The model under review builds one solid part; all positions refer to its coordinate system, in mm. A direction names the side the tool comes from. Round coordinates to 2 decimals unless told otherwise and drop trailing zeros. Write each loop counter-clockwise with the first axis right and the second up, starting at its lowest first coordinate (ties: lowest second). Pieces come first, ordered by that corner, then holes.
Item 1: To check wall thickness, follow L1, parallel to X at y = -71, z = 66; L2, parallel to Y at x = 66.5, z = 15; L3, parallel to Z at x = -13, y = 63.5. State the ranges of each line that lie inside material, in increasing order.
Item 2: Add section B-B (x = 88). Give the boundary of the cut face in (y, z), plus the area to 3 significant figures.
Item 3: Clearance check with flat-ended pins moving along their axes: pin 1 Ø3 at (x, z) = (101.5, 70.5) entering from +Y; pin 2 Ø3 at (x, y) = (101.5, -36.5) entering from +Z; pin 3 Ø4 at (x, z) = (-59.5, 59.5) entering from +Y. State where each tip first meets the part, or that it passes through.
Item 4: Add section C-C (z = 49). Give the boundary of the cut face in (x, y), plus the area to 3 significant figures.
Item 5: Machinability: for faces 1 (the face through (59.73, -48.19, 1.27)), 2 (the face through (101.871, -55.646, 56.504)), 3 (the face through (98.35, -95.36, 42.96)), which of the approach directions +Z, -Z, +X, -X, +Y, -Y give a long, thin tool a straight path to every point of the face, cutting with its end or side? Answer none if there is none.
Item 6: Add section D-D (y = -19). Give the boundary of the cut face in (x, z), plus the area to 3 significant figures.
Item 7: Draft analysis for pull direction X (two halves, no side actions). For faces 4 (the face through (100.603, -1, 42)), 5 (the face through (-93.89, -19.02, 2.85)), 6 (the face through (100.096, -1.26, 2.852)), state which applies: +X half, -X half, draft (parallel to the pull), parting line (faces both ways), or undercut.
Item 8: Add section A-A (z = 15). Give the boundary of the cut face in (x, y), plus the area to 3 significant figures.
```python
from build123d import *

# Parameters (mm, degrees)
F0_W      = 200
F0_H      = 200
F1_DEPTH  = 75
F2_R      = 10
F3_R      = 50
F4_R      = 10
F5_T      = -2.5
F6_R      = 20.601636
F7_DEPTH  = 200.001
F9_DEPTH  = 2.5
F11_DEPTH = 2.5


with BuildPart() as f1:
    # F0 (on Top) → F1 (new body)
    with BuildSketch(Plane.XY):
        with Locations((3.103165, 0)):
            Rectangle(F0_W, F0_H)
    extrude(amount=F1_DEPTH)

    # F2
    f2_edges = [f1.edges().sort_by_distance(p)[0] for p in [
        (-96.896835, -100, 37.5),
        (103.103165, -100, 37.5),
        (103.103165, 100, 37.5),
    ]]
    fillet(f2_edges, radius=F2_R)

    # F3
    f3_edges = [f1.edges().sort_by_distance(p)[0] for p in [
        (-96.896835, 100, 37.5),
    ]]
    fillet(f3_edges, radius=F3_R)

    # F4
    f4_edges = [f1.edges().sort_by_distance(p)[0] for p in [
        (23.103165, 100, 0),
    ]]
    fillet(f4_edges, radius=F4_R)

    # F5
    f5_openings = [f1.faces().sort_by_distance(p)[0] for p in [
        (4.259549, -1.156383, 75),
    ]]
    offset(amount=F5_T, openings=f5_openings)

    # F6 (on face) → F7 (cut, through all)
    with BuildSketch(Plane.XZ.offset(100)):
        with Locations((0, 44.865675)):
            Circle(F6_R)
    extrude(amount=-F7_DEPTH, mode=Mode.SUBTRACT)

    # F8 (on face) → F9 (cut, through all)
    with BuildSketch(Plane.XY.offset(2.5)):
        with BuildLine():
            ThreePointArc((54.924048, -7.537108), (51.811896, -2.99646), (50.547384, 2.361149))
            ThreePointArc((50.547384, 2.361149), (-39.923575, 29.284524), (14.04054, -48.160533))
            ThreePointArc((14.04054, -48.160533), (21.879419, -48.100018), (28.678354, -52.002092))
            Line((28.678354, -52.002092), (42.298151, -65.621889))
            Line((42.298151, -65.621889), (77.65349, -30.26655))
            Line((77.65349, -30.26655), (54.924048, -7.537108))
        make_face()
    extrude(amount=-F9_DEPTH, mode=Mode.SUBTRACT)

    # F10 (on face) → F11 (cut, through all)
    with BuildSketch(Plane.YZ.offset(103.103165)):
        with BuildLine():
            ThreePointArc((-57.071527, 60), (-55.607061, 56.464466), (-52.071527, 55))
            Line((-52.071527, 55), (-5, 55))
            ThreePointArc((-5, 55), (-1.464466, 56.464466), (0, 60))
            Line((0, 60), (0, 75))
            Line((0, 75), (-57.071527, 75))
            Line((-57.071527, 75), (-57.071527, 60))
        make_face()
    extrude(amount=-F11_DEPTH, mode=Mode.SUBTRACT)


solid = f1.part
```
Numbers:
1. L1: x = -96.9 to -94.4, 100.6 to 103.1
1. L2: y = -100 to -97.5, 97.5 to 100
1. L3: z = 0 to 2.5
2. outline: (-100, 10) arc R10 ccw to (-90, 0) - (90, 0) arc R10 ccw to (100, 10) - (100, 75) - (97.5, 75) - (97.5, 10) arc R7.5 cw to (90, 2.5) - (-90, 2.5) arc R7.5 cw to (-97.5, 10) - (-97.5, 75) - (-100, 75) - close
2. area: 844 mm2
3. pin 1: stops at y = 97.24
3. pin 2: stops at z = 55
3. pin 3: stops at y = 98.86
4. outline: (-96.9, -90) arc R10 ccw to (-86.9, -100) - (-20.18, -100) - (-20.18, -97.5) - (-86.9, -97.5) arc R7.5 cw to (-94.4, -90) - (-94.4, 50) arc R47.5 cw to (-46.9, 97.5) - (-20.18, 97.5) - (-20.18, 100) - (-46.9, 100) arc R50 ccw to (-96.9, 50) - close; (20.18, -100) - (93.1, -100) arc R10 ccw to (103.1, -90) - (103.1, 90) arc R10 ccw to (93.1, 100) - (20.18, 100) - (20.18, 97.5) - (93.1, 97.5) arc R7.5 cw to (100.6, 90) - (100.6, -90) arc R7.5 cw to (93.1, -97.5) - (20.18, -97.5) - close
4. area: 1,690 mm2
5. face 1: +Z, -Z
5. face 2: +Z, +X
5. face 3: +Z
6. outline: (-96.9, 10) arc R10 ccw to (-86.9, 0) - (-45.65, 0) - (-45.65, 2.5) - (-86.9, 2.5) arc R7.5 cw to (-94.4, 10) - (-94.4, 75) - (-96.9, 75) - close; (66.39, 0) - (93.1, 0) arc R10 ccw to (103.1, 10) - (103.1, 55) - (100.6, 55) - (100.6, 10) arc R7.5 cw to (93.1, 2.5) - (66.39, 2.5) - close
6. area: 514 mm2
7. face 4: undercut
7. face 5: -X half
7. face 6: +X half
8. outline: (-96.9, -90) arc R10 ccw to (-86.9, -100) - (93.1, -100) arc R10 ccw to (103.1, -90) - (103.1, 90) arc R10 ccw to (93.1, 100) - (-46.9, 100) arc R50 ccw to (-96.9, 50) - close; hole (-94.4, -90) arc R7.5 ccw to (-86.9, -97.5) - (93.1, -97.5) arc R7.5 ccw to (100.6, -90) - (100.6, 90) arc R7.5 ccw to (93.1, 97.5) - (-46.9, 97.5) arc R47.5 ccw to (-94.4, 50) - close
8. area: 1,890 mm2
